Build history of the part. All positions in model axes, mm. A direction names the side the tool comes from. Round coordinates to 2 decimals unless told otherwise and drop trailing zeros. Loops run counter-clockwise (first coordinate to the right, second up) from the corner with the lowest first, then second, coordinate; pieces in that order, holes last. Notation, with made-up numbers: (28, -10.5) - (34, -10.5) arc R20 ccw to (34, 23.5) - close; hole circle Ø8 at (5, -20). An arc over 180 degrees is marked (long way). Use a Markdown table: item, result.
from build123d import *

# Parameters (mm, degrees)
F1_DEPTH      = 17
F3_DEPTH      = 150
F3_DEPTH_BACK = 25


with BuildPart() as f1:
    # F0 (on Top) → F1 (new body)
    with BuildSketch(Plane.XY):
        with BuildLine():
            Line((-11.8825086199, -21.935047995), (-8.9312226237, -22.4734818057))
            Line((-8.9312226237, -22.4734818057), (-8.213310876, -18.5384338107))
            ThreePointArc((-8.213310876, -18.5384338107), (-9.4197369687, -16.7935739073), (-11.1645968722, -18))
            Line((-11.1645968722, -18), (-11.8825086199, -21.935047995))
        make_face()
        with BuildLine():
            ThreePointArc((2.6638383122, 27.5), (3.7969927434, 29.2933099796), (5.5903028117, 28.1601556887))
            ThreePointArc((5.5903028117, 28.1601556887), (11.8707301214, 0.3190753529), (3.0978968201, -26.8398443113))
            ThreePointArc((3.0978968201, -26.8398443113), (-0.908917448, -29.8768455436), (-5.8834154579, -29.1472520849))
            Line((-5.8834154579, -29.1472520849), (-7.4091766717, -31.7302837762))
            ThreePointArc((-7.4091766717, -31.7302837762), (-0.162444822, -32.7824020899), (5.6797630841, -28.3675768125))
            ThreePointArc((5.6797630841, -28.3675768125), (14.8647434728, 0.183397229), (8.2997657894, 29.4481038135))
            ThreePointArc((8.2997657894, 29.4481038135), (3.1422456973, 32.1957980128), (-0.3361616878, 27.5))
            Line((-0.3361616878, 27.5), (-0.3361616878, 26))
            ThreePointArc((-0.3361616878, 26), (1.1638383122, 24.5), (2.6638383122, 26))
            Line((2.6638383122, 26), (2.6638383122, 27.5))
        make_face()
        with BuildLine():
            Line((-10.5465240559, -31.3273397943), (-10.1639891219, -29.2305732632))
            ThreePointArc((-10.1639891219, -29.2305732632), (-11.7731559311, -25.7594572525), (-11.8825086199, -21.935047995))
            Line((-11.8825086199, -21.935047995), (-12.3404061236, -24.444895006))
            Line((-12.3404061236, -24.444895006), (-13.7607384363, -32.2300800757))
            Line((-13.7607384363, -32.2300800757), (-5.4662183221, -41.5347142683))
            ThreePointArc((-5.4662183221, -41.5347142683), (-3.3483834547, -41.6562686781), (-3.2268290449, -39.5384338107))
            Line((-3.2268290449, -39.5384338107), (-10.5465240559, -31.3273397943))
        make_face()
        with BuildLine():
            Line((-7.4091766717, -31.7302837762), (-5.8834154579, -29.1472520849))
            ThreePointArc((-5.8834154579, -29.1472520849), (-8.4389300147, -26.2814876442), (-8.9312226237, -22.4734818057))
            Line((-8.9312226237, -22.4734818057), (-10.1639891219, -29.2305732632))
            ThreePointArc((-10.1639891219, -29.2305732632), (-8.9101299966, -30.6165839213), (-7.4091766717, -31.7302837762))
        make_face()
        with BuildLine():
            Line((-10.1639891219, -29.2305732632), (-8.9312226237, -22.4734818057))
            Line((-8.9312226237, -22.4734818057), (-11.8825086199, -21.935047995))
            ThreePointArc((-11.8825086199, -21.935047995), (-11.7731559311, -25.7594572525), (-10.1639891219, -29.2305732632))
        make_face()
    extrude(amount=F1_DEPTH)

    # F2 (on Right) → F3 (cut, two sides)
    with BuildSketch(Plane.YZ) as f3_sk:
        Polygon((49.3275342038, 11.2), (28.4481038135, 11.2), (14.4481038135, 11.2), (14.4481038135, 5.8), (49.3275342038, 5.8), align=None)
    extrude(amount=-F3_DEPTH, mode=Mode.SUBTRACT)
    extrude(f3_sk.sketch, amount=F3_DEPTH_BACK, mode=Mode.SUBTRACT)


solid = f1.part
Q1. Cut at C-C, the plane y = 1. List the corners of the cut face in (x, z), plus the area to 3 significant figures.
Results found:
| item | result |
|---|---|
| outline | (11.9, 0) - (14.9, 0) - (14.9, 17) - (11.9, 17) - close |
| area | 51.0 mm2 |
Q2. Which spindle directions (+Z, -Z, +X, -X, +Y, -Y) get a long thin tool onto all of the face, cutting with end or side? Do faces 1 (the face through (12, 14.448, 9)), 2 (the face through (1.1, 24.5, 14.1)), 3 (the face through (11.14, -7.45, 0)). Say none if no direction does.
Results found:
| item | result |
|---|---|
| face 1 | +X, -X, +Y |
| face 2 | +Z, -Z |
| face 3 | -Z, +X, -X, +Y, -Y |
Q3. Drop flat-ended pins along their axis: pin 1 (3.5 mm diameter, centred on x = 12.5, z = 8.5, fed in from +Y); pin 2 (0.8 mm diameter, centred on y = 27, z = 2, fed in from +X); pin 3 (1 mm diameter, centred on y = 18, z = 14, fed in from +X). Give the stop position or say it passes through.
Results found:
| item | result |
|---|---|
| pin 1 | stops at y = 14.45 |
| pin 2 | stops at x = 9.71 |
| pin 3 | stops at x = 12.99 |
Q4. Cut at D-D, the plane y = 11. List the corners of the cut face in (x, z), plus the area to 3 significant figures.
Results found:
| item | result |
|---|---|
| outline | (11.3, 0) - (14.33, 0) - (14.33, 17) - (11.3, 17) - close |
| area | 51.5 mm2 |
Q5. Pull direction Z, two halves, no side cores. Call faces 4 (the face through (11.14, -7.45, 17)), 5 (the face through (7.2, 25.3, 5.8)), 6 (the face through (3.765, 29.286, 2.859)): pulls with the +Z half, pulls with the -Z half, needs draft (parallel to the pull), parting line crosses it, or undercut.
Results found:
| item | result |
|---|---|
| face 4 | pulls with the +Z half |
| face 5 | undercut |
| face 6 | needs draft |
Q6. Cut at A-A, the plane z = 13.5. List the corners of the cut face in (x, y), plus the area to 3 significant figures.
Results found:
| item | result |
|---|---|
| outline | (-13.76, -32.23) - (-5.47, -41.53) arc R1.5 ccw to (-3.23, -39.54) - (-10.55, -31.33) - (-10.16, -29.23) arc R9.5 ccw to (5.68, -28.37) arc R57.05 ccw to (8.3, 29.45) arc R4.48 ccw to (-0.34, 27.5) - (-0.34, 26) arc R1.5 ccw to (2.66, 26) - (2.66, 27.5) arc R1.5 cw to (5.59, 28.16) arc R54.06 cw to (3.1, -26.84) arc R6.5 cw to (-8.93, -22.47) - (-8.21, -18.54) arc R1.5 ccw to (-11.16, -18) - close |
| area | 348 mm2 |
Q7. Cut at B-B, the plane x = 4.5. List the corners of the cut face in (y, z).
Results found:
| item | result |
|---|---|
| outline | (-29.97, 0) - (-24.58, 0) - (-24.58, 17) - (-29.97, 17) - close; (29.28, 0) - (32.29, 0) - (32.29, 5.8) - (29.28, 5.8) - close; (29.28, 11.2) - (32.29, 11.2) - (32.29, 17) - (29.28, 17) - close |
Q8. Probe line 1 (X direction, y = -22, z = 7.25); line 2 (Y direction, x = -8, z = 15); line 3 (Y direction, x = 6.5, z = 1.5). List the from-to ranges inside material, lowest first.
Results found:
| item | result |
|---|---|
| line 1 | x = -11.89 to -8.84, 5.92 to 9.27 |
| line 2 | y = -38.69 to -34.18, -31.35 to -27.09 |
| line 3 | y = -27.07 to -20.84, 26.37 to 31.62 |
